```python
from build123d import *

# Parameters (mm, degrees)
BOSS_EXTRUDE1_DEPTH                                 = 15.875
SKETCH3_W                                           = 25.4
SKETCH3_H                                           = 12.7
CUT_EXTRUDE1_DEPTH                                  = 33.534068682
F_10_CLEARANCE_HOLE1_D                              = 5.1054
CBORE_FOR_10_BINDING_HEAD_MACHINE_SCREW_D           = 5.1054
CBORE_FOR_10_BINDING_HEAD_MACHINE_SCREW_CBORE_D     = 11.1125
CBORE_FOR_10_BINDING_HEAD_MACHINE_SCREW_CBORE_DEPTH = 3.1242


with BuildPart() as part:
    # Sketch1 → Boss-Extrude1 (new, symmetric)
    with BuildSketch(Plane.XY):
        with BuildLine():
            Line((-12.7, 0), (-12.7, -12.7))
            Line((-12.7, -12.7), (12.7, -12.7))
            Line((12.7, -12.7), (12.7, 0))
            ThreePointArc((12.7, 0), (0, 12.7), (-12.7, 0))
        make_face()
    extrude(amount=BOSS_EXTRUDE1_DEPTH, both=True)

    # Sketch3 → Cut-Extrude1 (cut, through all)
    with BuildSketch(Plane(origin=(12.7, 0, 0), x_dir=(0, 0, -1), z_dir=(1, 0, 0))):
        with Locations((0, 6.35)):
            Rectangle(SKETCH3_W, SKETCH3_H)
    extrude(amount=-CUT_EXTRUDE1_DEPTH, mode=Mode.SUBTRACT)

    # #10 Clearance Hole1 (through all)
    with Locations(Plane.XY.offset(15.875)):
        with Locations((0, 6.35)):
            Hole(F_10_CLEARANCE_HOLE1_D / 2)

    # CBORE for #10 Binding Head Machine Screw1 (through all)
    with Locations(Plane(origin=(0, 0, 0), x_dir=(1, 0, 0), z_dir=(0, 1, 0))):
        with Locations((0, 0)):
            CounterBoreHole(CBORE_FOR_10_BINDING_HEAD_MACHINE_SCREW_D / 2, CBORE_FOR_10_BINDING_HEAD_MACHINE_SCREW_CBORE_D / 2, CBORE_FOR_10_BINDING_HEAD_MACHINE_SCREW_CBORE_DEPTH)


solid = part.part
```
Could you check a few things on this model? Use its own coordinates, in mm. A direction names the side the tool comes from. Coordinates: 2 decimals unless noted, no trailing zeros. Write each loop counter-clockwise with the first axis right and the second up, starting at its lowest first coordinate (ties: lowest second). Pieces come first, ordered by that corner, then holes. Notation, with made-up numbers: (-6.5, -9) -> (41.5, -9) arc R8 cw to (41.5, -2) -> close; hole circle Ø3 at (21, -31). An arc over 180 degrees is marked (long way). One line per question, with ' | ' between items. Start each with the question number.
1. Thinking about a two-plate mould opening in X: for faces 4 (the face through (0.279, 12.697, 14.31)), 5 (the face through (1, 4, -14)), 6 (the face through (0, 3, 12.7)), which applies, pulls with the +X half, pulls with the -X half, needs draft (parallel to the pull), parting line crosses it, or undercut?
2. For faces 1 (the face through (0, 3, -12.7)), 2 (the face through (-1.3, -3.124, 2.4)), 3 (the face through (12.7, -6, 0)), which set-ups out of +Z, -Z, +X, -X, +Y, -Y let a thin tool reach every point of the face, with its end or its side?
3. If we section it at C-C (y = -11): Please give me the cut outline in (x, z) (3 decimals), and give its area (3 significant figures).
4. If we section it at B-B (x = 0): Please give me the cut outline in (y, z) (3 decimals), and give its area (3 significant figures).
5. Please list where these lines run through material, in increasing order: line 1 along Z through (x, y) = (6.25, 5) (3 decimals); line 2 along Y through (x, z) = (0, -14.05); line 3 along Z through (x, y) = (0, -1) (3 decimals).
6. If we section it at D-D (y = 6.35): Please give me the cut outline in (x, z) (3 decimals).
7. Will these pins go through, and if not, where does the flat tip stop? P1, Ø9, axis at x = 0, z = 0, coming from the +Y side; P2, Ø8, axis at x = 1, y = 7.5, coming from the -Z side (3 decimals); P3, Ø10, axis at x = 7.5, z = 11.5, coming from the +Y side; P4, Ø12, axis at x = -1, z = 0.5, coming from the +Y side.
8. If we section it at A-A (z = 0): Please give me the cut outline in (x, y), and give its area (3 significant figures).
Return value:
1) face 4: parting line crosses it | face 5: undercut | face 6: needs draft
2) face 1: +X, -X, +Y | face 2: +Y | face 3: +Z, -Z, +X, +Y, -Y
3) outline: (-12.7, -15.875) -> (12.7, -15.875) -> (12.7, 15.875) -> (-12.7, 15.875) -> close; hole circle Ø5.105 at (0, 0) | area: 786 mm²
4) outline: (-12.7, -15.875) -> (3.797, -15.875) -> (3.797, -12.7) -> (0, -12.7) -> (0, -5.556) -> (-3.124, -5.556) -> (-3.124, -2.553) -> (-12.7, -2.553) -> close; (-12.7, 2.553) -> (-3.124, 2.553) -> (-3.124, 5.556) -> (0, 5.556) -> (0, 12.7) -> (3.797, 12.7) -> (3.797, 15.875) -> (-12.7, 15.875) -> close; (8.903, -15.875) -> (12.7, -15.875) -> (12.7, -12.7) -> (8.903, -12.7) -> close; (8.903, 12.7) -> (12.7, 12.7) -> (12.7, 15.875) -> (8.903, 15.875) -> close | area: 368 mm²
5) line 1: z = -15.875 to -12.7, 12.7 to 15.875 | line 2: y = -12.7 to 3.8, 8.9 to 12.7 | line 3: z = -15.875 to -5.556, 5.556 to 15.875
6) outline: (-10.999, -15.875) -> (-2.553, -15.875) -> (-2.553, -12.7) -> (-10.999, -12.7) -> close; (-10.999, 12.7) -> (-2.553, 12.7) -> (-2.553, 15.875) -> (-10.999, 15.875) -> close; (2.553, -15.875) -> (10.999, -15.875) -> (10.999, -12.7) -> (2.553, -12.7) -> close; (2.553, 12.7) -> (10.999, 12.7) -> (10.999, 15.875) -> (2.553, 15.875) -> close
7) P1: stops at y = -3.12 | P2: stops at z = -15.875 | P3: stops at y = 12.42 | P4: stops at y = 0
8) outline: (-12.7, -12.7) -> (-2.55, -12.7) -> (-2.55, -3.12) -> (-5.56, -3.12) -> (-5.56, 0) -> (-12.7, 0) -> close; (2.55, -12.7) -> (12.7, -12.7) -> (12.7, 0) -> (5.56, 0) -> (5.56, -3.12) -> (2.55, -3.12) -> close | area: 239 mm²
